Can you work these out from the drawing? Everything is in mm from the part's minimum corner. A direction names the side the tool comes from. Coordinates: 2 decimals unless noted, no trailing zeros. Write each loop counter-clockwise with the first axis right and the second up, starting at its lowest first coordinate (ties: lowest second). Pieces come first, ordered by that corner, then holes.
(1) Thinking about a two-plate mould opening in Z: for the marked faces 4, 5 and 6, which applies, released by +Z, released by -Z, zero draft, split by the parting line, or undercut?
(2) Imagine slicing it at D-D, the plane y = 10. List the corners of the cut face in (x, z) for me.
(3) Imagine slicing it at C-C, the plane z = 5. List the corners of the cut face in (x, y) for me.
(4) Imagine slicing it at B-B, the plane x = 5. List the corners of the cut face in (y, z) for me, plus the area to 3 significant figures.
(5) For pin 1 Ø3.5 at (x, z) = (26, 5) entering from +Y; pin 2 Ø2 at (x, z) = (7, 3.5) entering from -Y; pin 3 Ø1 at (x, z) = (14.5, 9) entering from -Y, each with a flat end and sliding along its axis, tell me the tip position at first contact or that it passes through.
(6) Which directions (+Z, -Z, +X, -X, +Y, -Y) give clear straight access to the entire face, cutting with the end or side of a thin tool? Please do the marked faces 1, 2 and 3.
(7) Please list where these lines run through material, in increasing order: probe 1 along X at (y, z) = (10, 5.5); probe 2 along X at (y, z) = (10, 4); probe 3 along X at (y, z) = (2.5, 4).
(8) Imagine slicing it at A-A, the plane y = 8. List the corners of the cut face in (x, z) for me, plus the area to 3 significant figures.
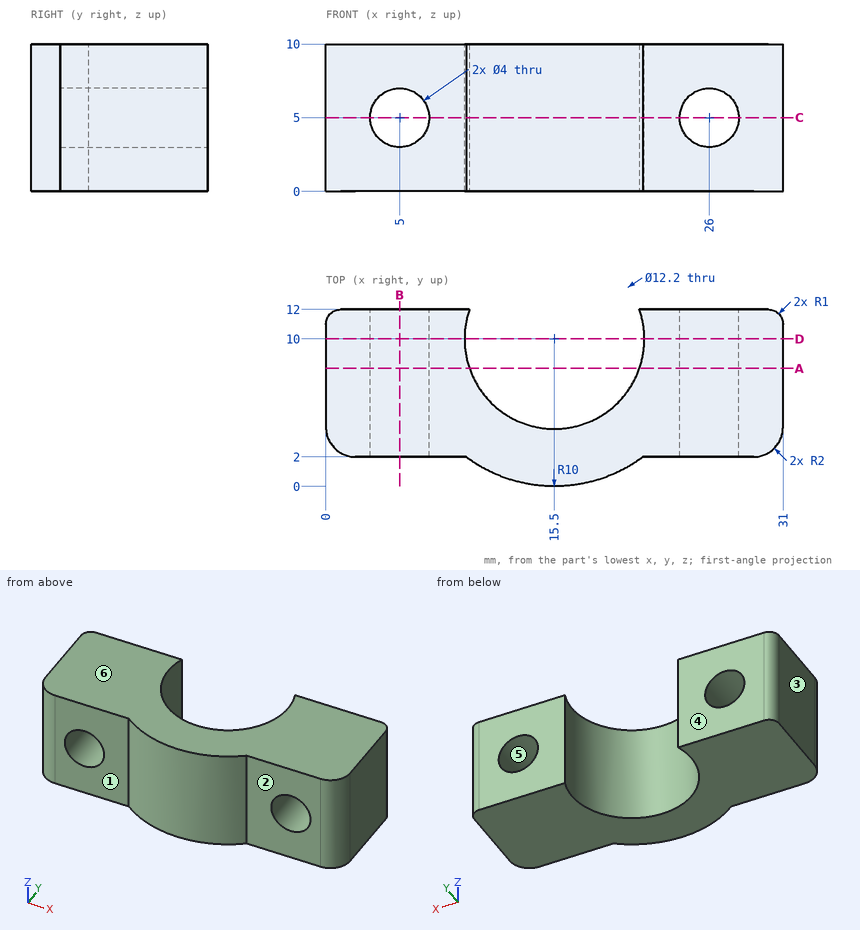
Recorded:
1. face 4: zero draft
1. face 5: undercut
1. face 6: released by +Z
2. outline: (0, 0) - (9.4, 0) - (9.4, 10) - (0, 10) - close; (21.6, 0) - (31, 0) - (31, 10) - (21.6, 10) - close; hole circle Ø4 at (5, 5); hole circle Ø4 at (26, 5)
3. outline: (0, 4) arc R2 ccw to (2, 2) - (3, 2) - (3, 12) - (1, 12) arc R1 ccw to (0, 11) - close; (7, 2) - (9.5, 2) arc R10 ccw to (21.5, 2) - (24, 2) - (24, 12) - (21.26, 12) arc R6.1 cw (long way) to (9.74, 12) - (7, 12) - close; (28, 2) - (29, 2) arc R2 ccw to (31, 4) - (31, 11) arc R1 ccw to (30, 12) - (28, 12) - close
4. outline: (2, 0) - (12, 0) - (12, 3) - (2, 3) - close; (2, 7) - (12, 7) - (12, 10) - (2, 10) - close
4. area: 60.0 mm2
5. pin 1: passes through
5. pin 2: stops at y = 2
5. pin 3: stops at y = 0.01
6. face 1: +Z, -Z, -X, -Y
6. face 2: +Z, -Z, +X, -Y
6. face 3: +Z, -Z, -X, +Y, -Y
7. probe 1: x = 0 to 3.06, 6.94 to 9.4, 21.6 to 24.06, 27.94 to 31
7. probe 2: x = 0 to 3.27, 6.73 to 9.4, 21.6 to 24.27, 27.73 to 31
7. probe 3: x = 0.68 to 3.27, 6.73 to 24.27, 27.73 to 30.32
8. outline: (0, 0) - (9.74, 0) - (9.74, 10) - (0, 10) - close; (21.26, 0) - (31, 0) - (31, 10) - (21.26, 10) - close; hole circle Ø4 at (5, 5); hole circle Ø4 at (26, 5)
8. area: 170 mm2
